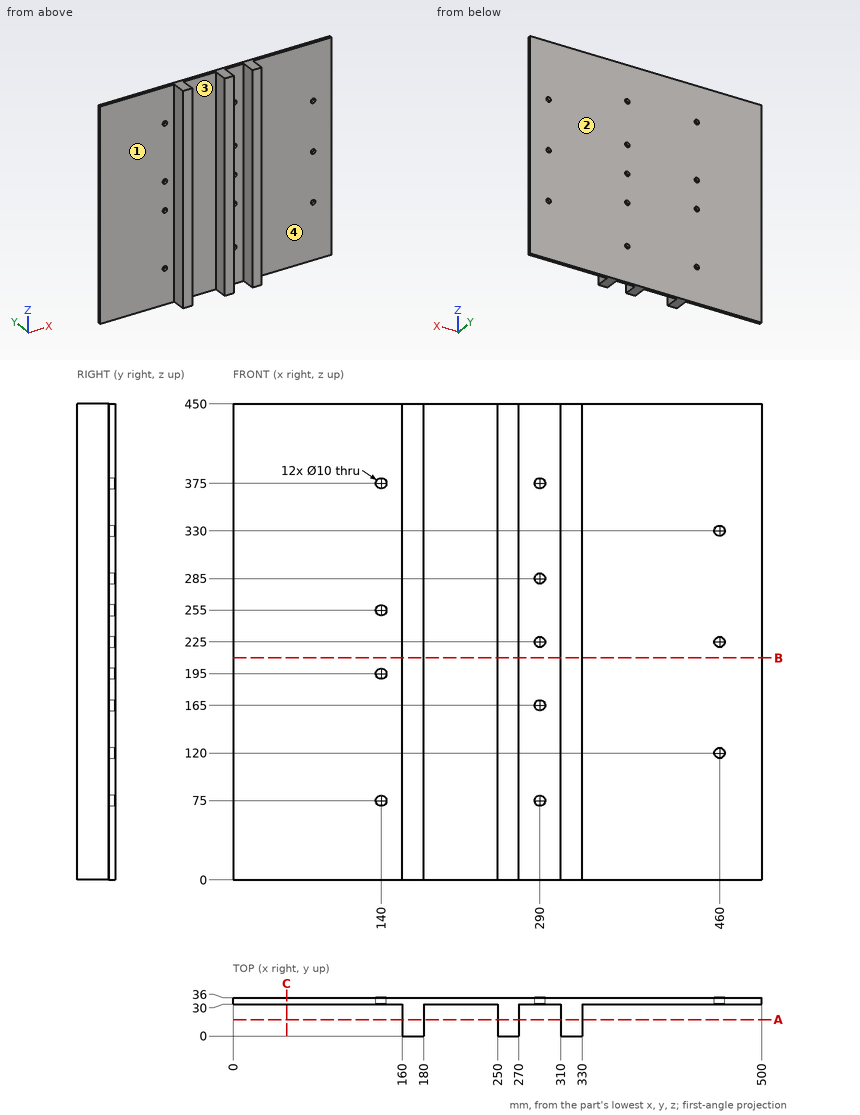
Print and shaded views of the part. All mm, measured from the part's lowest x, y and z. A direction names the side the tool comes from. Coordinates: 2 decimals unless noted, no trailing zeros. Order: outer loops, then holes, each group sorted by start corner. A loop starts at its lowest first (then second) coordinate and runs counter-clockwise, first axis right, second up. Notation, with made-up numbers: (82, 65.25) -> (140, 65.25) arc R18 cw to (140, 80.25) -> close; hole circle Ø8 at (69, -28). An arc over 180 degrees is marked (long way). Use one line per item in the form item = value. Start each with the question number.
1) Band-saw the part on C-C on x = 50.5. Give the cut face in (y, z).
2) Pull direction X, two halves, no side cores. Call the marked faces 3 and 4: +X half, -X half, draft (parallel to the pull), parting line (faces both ways), or undercut.
3) Band-saw the part on A-A on y = 15.5. Give the cut face in (x, z).
4) Drill centre lines: L1, parallel to X at y = 34, z = 225; L2, parallel to Z at x = 290, y = 32; L3, parallel to X at y = 19, z = 121.5. Where is each one in solid material? Low to high. Write a range as [from, to].
5) Drop flat-ended pins along their axis: pin 1 (4 mm diameter, centred on y = 23.5, z = 79.5, fed in from +X); pin 2 (2 mm diameter, centred on x = 285.5, z = 216, fed in from -Y); pin 3 (5 mm diameter, centred on y = 15, z = 118, fed in from -X). Give the stop position or say it passes through.
6) Band-saw the part on B-B on z = 210. Give the cut face in (x, y), then the cut area to 3 significant figures.
7) Tool access for the marked faces 1 and 2: list every direction of +Z, -Z, +X, -X, +Y, -Y with a clear straight run to the whole face (end or side of a thin tool).
Entries:
q1.outline = (30, 0) -> (36, 0) -> (36, 450) -> (30, 450) -> close
q2.face_3 = undercut
q2.face_4 = draft
q3.outline = (160, 0) -> (180, 0) -> (180, 450) -> (160, 450) -> close; (250, 0) -> (270, 0) -> (270, 450) -> (250, 450) -> close; (310, 0) -> (330, 0) -> (330, 450) -> (310, 450) -> close
q4.L1 = [0, 285], [295, 455], [465, 500]
q4.L2 = [0, 70], [80, 160], [170, 220], [230, 280], [290, 370], [380, 450]
q4.L3 = [160, 180], [250, 270], [310, 330]
q5.pin_1 = 330
q5.pin_2 = 30
q5.pin_3 = 160
q6.outline = (0, 30) -> (160, 30) -> (160, 0) -> (180, 0) -> (180, 30) -> (250, 30) -> (250, 0) -> (270, 0) -> (270, 30) -> (310, 30) -> (310, 0) -> (330, 0) -> (330, 30) -> (500, 30) -> (500, 36) -> (0, 36) -> close
q6.area = 4,800 mm2
q7.face_1 = +Z, -Z, -X, -Y
q7.face_2 = +Z, -Z, +X, -X, +Y
